from build123d import *

# Parameters (mm, degrees)
F2_W          = 63.5
F2_H          = 14.5669
F3_DEPTH      = 3.81
F3_DEPTH_BACK = 3.81
F5_DEPTH      = 18.0985
F10_W         = 203.2
F10_H         = 3.175


with BuildPart() as f1:
    # F0 (on Front) → F1 (revolve)
    with BuildSketch(Plane.XZ):
        Polygon((148.59, 0), (148.59, 14.2875), (81.28, 12.7), (81.28, 9.2075), (63.5, 9.2075), (63.5, 6.096), (0, 6.096), (0, 0), align=None)
    revolve(axis=Axis((74.295, 0, 0), (1, 0, 0)))

    # F2 (on Front) → F3 (join, two sides)
    with BuildSketch(Plane.XZ) as f3_sk:
        with Locations((31.75, -7.28345)):
            Rectangle(F2_W, F2_H)
    extrude(amount=F3_DEPTH)
    extrude(f3_sk.sketch, amount=-F3_DEPTH_BACK)

    # F4 (on face) → F5 (cut, through all)
    with BuildSketch(Plane.XZ.offset(3.81)):
        Polygon((14.1605, -7.62), (7.62, -14.5669), (15.875, -14.5669), (15.875, -7.62), align=None)
        Polygon((15.875, -7.62), (15.875, -14.5669), (24.13, -14.5669), (17.5895, -7.62), align=None)
    extrude(amount=-F5_DEPTH, mode=Mode.SUBTRACT)

    # F6 (on Front) → F9 (revolve)
    with BuildSketch(Plane.XZ):
        with BuildLine():
            Line((148.59, 0), (162.8775, 0))
            ThreePointArc((162.8775, 0), (158.692788, 10.102788), (148.59, 14.2875))
            Line((148.59, 14.2875), (148.59, 0))
        make_face()
    revolve(axis=Axis((155.73375, 0, 0), (1, 0, 0)))

    # F10 (on Front) → F11 (revolve)
    with BuildSketch(Plane.XZ):
        with Locations((76.2, 1.5875)):
            Rectangle(F10_W, F10_H)
    revolve(axis=Axis((76.2, 0, 0), (1, 0, 0)))


with BuildPart() as f7:
    # F6 (on Front) → F7 (revolve)
    with BuildSketch(Plane.XZ):
        with BuildLine():
            Line((148.59, 0), (162.8775, 0))
            ThreePointArc((162.8775, 0), (158.692788, 10.102788), (148.59, 14.2875))
            Line((148.59, 14.2875), (148.59, 0))
        make_face()
    revolve(axis=Axis((155.73375, 0, 0), (-1, 0, 0)))


solid = f1.part
Verification items for the finished model (mm, model axes). A direction names the side the tool comes from. Round coordinates to 2 decimals unless told otherwise and drop trailing zeros. Order: outer loops, then holes, each group sorted by start corner. A loop starts at its lowest first (then second) coordinate and runs counter-clockwise, first axis right, second up.
1. Section check C-C on x = -9.5. Record the cut outline in (y, z) (3 decimals).
Final values:
outline: circle Ø6.35 at (0, 0)
2. Section check B-B on x = 29.5. Record the cut outline in (y, z).
Final values:
outline: (-3.81, -14.57) - (3.81, -14.57) - (3.81, -4.76) arc R6.1 ccw (long way) to (-3.81, -4.76) - close
3. Access from +Z, -Z, +X, -X, +Y, -Y to the whole of each face (thin tool, end or side, straight path). Record for faces 1 (the cylindrical face through (170.27, 3.1, -0.69)), 2 (the flat face through (81.28, -7, 7)), 3 (the flat face through (10.94, -0.05, -11.04)), 4 (the flat face through (63.5, 2, 6)).
Final values:
face 1: +X
face 2: none
face 3: -Z, +Y, -Y
face 4: -X
4. Release check for a two-part mould opening along X. For faces 5 (the flat face through (-25.4, 0, 0)), 6 (the flat face through (31, 3.81, -10)), 7 (the flat face through (20.906, -0.053, -11.142)) record: +X half, -X half, draft (parallel to the pull), parting line (faces both ways), or undercut.
Final values:
face 5: -X half
face 6: draft
face 7: undercut
5. Section check A-A on x = 70.5. Record the cut outline in (y, z) (1 decimal), then the cut area to 3 significant figures.
Final values:
outline: circle Ø18.4 at (0, 0)
area: 266 mm2
6. Thickness scan on L1, parallel to Z at x = 169, y = -0.25; L2, parallel to Y at x = 143, z = -6.25; L3, parallel to Y at x = 0.5, z = -10.75. Record the ranges inside material, lowest first.
Final values:
L1: z = -3.17 to 3.17
L2: y = -12.7 to 12.7
L3: y = -3.81 to 3.81
7. Go/stop test with flat-tipped pins: P1, Ø6, axis at x = 123.5, z = -0.5, coming from the +Y side; P2, Ø3, axis at y = -9.5, z = 3.5, coming from the -X side; P3, Ø5, axis at x = 29.5, z = -8.5, coming from the +Y side. Record where each tip stops, or that it passes through.
Final values:
P1: stops at y = 13.77
P2: stops at x = 63.5
P3: stops at y = 3.81
